Autodesk Inventor part; units mm, degrees
ref_plane "YZ Plane" through (0, 0, 0) normal (1, 0, 0) x (0, 1, 0)
ref_plane "XZ Plane" through (0, 0, 0) normal (0, 1, 0) x (-1, 0, 0)
ref_plane "XY Plane" through (0, 0, 0) normal (0, 0, 1) x (1, 0, 0)
sketch "Sketch1" plane through (0, 0, 0) normal (0, 0, 1) x (1, 0, 0)
  line L0 (2, 0) -> (20.9174, 0)
  line L1 (87, 2) -> (87, 54)
  line L2 (85, 56) -> (2, 56)
  line L3 (0, 54) -> (0, 2)
  line L4 (44.4174, 5) -> (44.4174, 0)
  arc A0 (2, 56) -> (0, 54) centre (2, 54) ccw
  arc A1 (87, 54) -> (85, 56) centre (85, 54) ccw
  arc A2 (85, 0) -> (87, 2) centre (85, 2) ccw
  arc A3 (0, 2) -> (2, 0) centre (2, 2) ccw
  line L5 (69.9174, 0) -> (85, 0)
  line L6 (20.9174, 0) -> (20.9174, 5)
  circle A4 centre (44.4174, 5) radius 23.5
  line L7 (67.9174, 0) -> (67.9174, 5)
  line L8 (67.9174, 0) -> (69.9174, 0)
  circle A5 centre (44.4174, 5) radius 25.5
  line L9 (18.9174, 5) -> (18.9174, 0)
  line L10 (69.9174, 5) -> (69.9174, 0)
  point P0 (0, 0)
  point P1 (87, 56)
  point P2 (87, 0)
  point P3 (0, 56)
  dimension "d0" = 87
  dimension "d1" = 56
  dimension "d2" = 5
  dimension "d7" = 2
  dimension "d10" = 20.9174
  dimension "d11" = 47
  dimension "d12" = 2
extrude "Extrusion1" add sketch "Sketch1" along normal blind 3 contours A3 L3 A0 L2 A1 L1 A2 L5 L10 A5 L9 L0
fillet "Fillet1" radius 2 2 edges at (18.9174, 0, 1.5) (69.9174, 0, 1.5)
sketch "Sketch2" plane through (0, 0, 3) normal (0, 0, 1) x (1, 0, 0)
  line L0 (4, 38) -> (16, 38)
  line L1 (16, 38) -> (16, 30)
  line L2 (16, 30) -> (4, 30)
  line L3 (4, 30) -> (4, 38)
  line L4 (2, 0) -> (16.9174, 0)
  line L5 (0, 54) -> (0, 2)
  circle A0 centre (8, 34) radius 4
  circle A1 centre (12, 34) radius 4
  point P0 (0, 0)
  point P1 (12, 38)
  point P2 (8, 38)
  point P3 (8, 30)
  point P4 (12, 30)
  dimension "d14" = 30
  dimension "d15" = 8
  dimension "d16" = 4
  dimension "d17" = 12
extrude "Extrusion2" cut sketch "Sketch2" against normal blind 3 contours L0 A1 A0 | A0 A1 | A1 A0 | A0 A1 | A0 A1 L2
properties part number "PAREDES LATERALES"
Source: CAD feature listing. Evaluate the final solid. Frame: model axes, mm. A direction names the side the tool comes from. Coordinates: 2 decimals unless noted, no trailing zeros. Loops run counter-clockwise (first coordinate to the right, second up) from the corner with the lowest first, then second, coordinate; pieces in that order, holes last. Notation, with made-up numbers: M 33.5,-19 L 59.5,-19 A24 ccw 59.5,12 Z; hole C 82.5,68 d3. An arc over 180 degrees is marked long. Use a Markdown table: item, result. Add a question column.
Q1. Section query A-A, the plane x = 10. Return loops of the section in (y, z), and give its area (3 significant figures).
Q2. Material intervals for L1, parallel to Y at x = 12, z = 1.9; L2, parallel to X at y = 27.5, z = 0.25; L3, parallel to X at y = 22, z = 1.8, sorted ascending.
Q3. Section query C-C, the plane z = 0.65. Return loops of the section in (x, y).
Q4. First-contact query: pin 1 (1 mm diameter, centred on x = 64.5, z = 1, fed in from -Y). Flat tip, straight axial feed; report the tip coordinate or a pass-through.
Q5. Section query D-D, the plane x = 63.5. Return loops of the section in (y, z).
Q6. Section query B-B, the plane y = 34. Return loops of the section in (x, z), and give its area (3 significant figures).
Q7. Access query for faces 4 (the flat face through (10, 38, 2)), 5 (the cylindrical face through (0.6, 0.57, 1.48)), 6 (the flat face through (18.917, 4, 1)). Directions: +Z, -Z, +X, -X, +Y, -Y. A direction counts if a zero-diameter tool reaches every point of the face in a straight line with its end or side. Return the directions, or none.
Q8. Draft query along Y for faces 1 (the cylindrical face through (70.49, 0.6, 1.52)), 2 (the flat face through (43, 35, 0)), 3 (the cylindrical face through (16, 34, 2)). Return one class per face: pulls with the +Y half, pulls with the -Y half, needs draft (parallel to the pull), parting line crosses it, or undercut.
Result:
| question | item | result |
|---|---|---|
| 1 | outline | M 0,0 L 30,0 L 30,3 L 0,3 Z; M 38,0 L 56,0 L 56,3 L 38,3 Z |
| 1 | area | 144 mm2 |
| 2 | L1 | y = 0 to 30, 38 to 56 |
| 2 | L2 | x = 0 to 32.42, 56.42 to 87 |
| 2 | L3 | x = 0 to 25.41, 63.42 to 87 |
| 3 | outline | M 0,2 A2 ccw 2,0 L 16.92,0 A2 ccw 18.92,2 L 18.92,5 A25.5 cw 69.92,5 L 69.92,2 A2 ccw 71.92,0 L 85,0 A2 ccw 87,2 L 87,54 A2 ccw 85,56 L 2,56 A2 ccw 0,54 Z; hole M 8,30 L 12,30 A4 ccw 12,38 L 8,38 A4 ccw Z |
| 4 | pin 1 | stops at y = 20.05 |
| 5 | outline | M 21.91,0 L 56,0 L 56,3 L 21.91,3 Z |
| 6 | outline | M 0,0 L 4,0 L 4,3 L 0,3 Z; M 16,0 L 87,0 L 87,3 L 16,3 Z |
| 6 | area | 225 mm2 |
| 7 | face 4 | +Z, -Z |
| 7 | face 5 | +Z, -Z, -X, -Y |
| 7 | face 6 | +Z, -Z, -Y |
| 8 | face 1 | pulls with the -Y half |
| 8 | face 2 | needs draft |
| 8 | face 3 | undercut |
